Geometry: final body of the model. Coordinates: model frame, mm. A direction names the side the tool comes from. Give positions to 0.01 mm unless a question says otherwise; leave off trailing zeros. Write each loop counter-clockwise with the first axis right and the second up, starting at its lowest first coordinate (ties: lowest second). Pieces come first, ordered by that corner, then holes. Notation, with made-up numbers: (-37, 22.25) -> (-15, 22.25) arc R26 ccw to (-15, 50.25) -> close; hole circle Ø7 at (36.5, 27.25). An arc over 180 degrees is marked (long way). Answer as a JSON object with one key per item and string values.
from build123d import *

# Parameters (mm, degrees)
EXTRUDE_1_DEPTH     = 3
CUT_EXTRUDE_1_DEPTH = 5
CUT_EXTRUDE_2_DEPTH = 5


with BuildPart() as part:
    # 草图1 → 凸台-拉伸1 (new body)
    with BuildSketch(Plane(origin=(0, 0, 0), x_dir=(1, 0, 0), z_dir=(0, 1, 0))):
        with BuildLine():
            Line((0, 50), (0, -50))
            ThreePointArc((0, -50), (-50, 0), (0, 50))
        make_face()
    extrude(amount=EXTRUDE_1_DEPTH)

    # 草图3 → 切除-拉伸1 (cut)
    with BuildSketch(Plane(origin=(0, 3, 0), x_dir=(1, 0, 0), z_dir=(0, 1, 0))):
        Polygon((-27.479570649, 27.155271417), (-10.562944149, 37.824280175), (-12.163295463, 40.36177415), (-29.079921962, 29.692765392), align=None)
        Polygon((-29.079921962, -29.692765392), (-27.479570649, -27.155271417), (-10.562944149, -37.824280175), (-12.163295463, -40.36177415), align=None)
    extrude(amount=-CUT_EXTRUDE_1_DEPTH, mode=Mode.SUBTRACT)

    # 草图4 → 切除-拉伸2 (cut)
    with BuildSketch(Plane(origin=(0, 3, 0), x_dir=(1, 0, 0), z_dir=(0, 1, 0))):
        Polygon((-29.442581692, -10), (-30, -10), (-30, -15), (-10, -15), (-10, -10), align=None)
    extrude(amount=-CUT_EXTRUDE_2_DEPTH, mode=Mode.SUBTRACT)


solid = part.part
Q1. Mould query, pull axis X, two halves, no side actions, for faces 3 (the flat face through (-19, 0, -1)), 4 (the flat face through (0, 1, -1)), 5 (the flat face through (-19.14, 1.521, -32.415)). Classes: pulls with the +X half, pulls with the -X half, needs draft (parallel to the pull), parting line crosses it, or undercut.
Values:
{"face 3": "needs draft", "face 4": "pulls with the +X half", "face 5": "undercut"}
Q2. Cut plane B-B (x = -23). Return the cut outline in (y, z), and give its area (3 significant figures).
Values:
{"outline": "(0, -44.4) -> (3, -44.4) -> (3, -33.53) -> (0, -33.53) -> close; (0, -29.98) -> (3, -29.98) -> (3, 10) -> (0, 10) -> close; (0, 15) -> (3, 15) -> (3, 29.98) -> (0, 29.98) -> close; (0, 33.53) -> (3, 33.53) -> (3, 44.4) -> (0, 44.4) -> close", "area": "230 mm²"}
Q3. Material intervals for L1, parallel to Z at x = -16, y = 2; L2, parallel to Z at x = -26, y = 2.2; L3, parallel to X at y = 1.55, z = -31, sorted ascending. Write a range as from..to.
Values:
{"L1": "-47.37..-37.94, -34.4..10, 15..34.4, 37.94..47.37", "L2": "-42.71..-31.64, -28.09..10, 15..28.09, 31.64..42.71", "L3": "-39.23..-27.01, -21.38..0"}
Q4. Cut plane C-C (x = -15). Return the cut outline in (y, z), and give its area (3 significant figures).
Values:
{"outline": "(0, -47.7) -> (3, -47.7) -> (3, -38.57) -> (0, -38.57) -> close; (0, -35.03) -> (3, -35.03) -> (3, 10) -> (0, 10) -> close; (0, 15) -> (3, 15) -> (3, 35.03) -> (0, 35.03) -> close; (0, 38.57) -> (3, 38.57) -> (3, 47.7) -> (0, 47.7) -> close", "area": "250 mm²"}
Q5. First-contact query: P1, Ø1.5, axis at x = -20.5, y = 1, coming from the -Z side; P2, Ø0.9, axis at x = -25, y = 1.5, coming from the +Z side. Flat tips, straight axial feed; report the tip coordinate or a pass-through.
Values:
{"P1": "z = -45.93", "P2": "z = 43.56"}
Q6. Cut plane D-D (z = 16). Return the cut outline in (x, y).
Values:
{"outline": "(-47.37, 0) -> (0, 0) -> (0, 3) -> (-47.37, 3) -> close"}
Q7. Set-up query: faces 1 (the flat face through (-20.503, 1.521, -35.102)), 2 (the flat face through (-19, 3, -1)). Return all of +Z, -Z, +X, -X, +Y, -Y with unobstructed straight access to the full face (end or side cutting, diameter ignored); none if empty.
Values:
{"face 1": "+Y, -Y", "face 2": "+Z, -Z, +X, -X, +Y"}
Q8. Cut plane A-A (y = 2.05). Return the cut outline in (x, z).
Values:
{"outline": "(0, -50) -> (0, 50) arc R50 ccw to start; hole (-30, 10) -> (-10, 10) -> (-10, 15) -> (-30, 15) -> close; hole (-29.08, -29.69) -> (-12.16, -40.36) -> (-10.56, -37.82) -> (-27.48, -27.16) -> close; hole (-29.08, 29.69) -> (-27.48, 27.16) -> (-10.56, 37.82) -> (-12.16, 40.36) -> close"}
